Autodesk Fusion 360 part; units mm, degrees
sketch "Sketch1" plane through (0, 0, 0) normal (0, 0, 1) x (1, 0, 0)
  line L0 (38.1, -38.1) -> (-38.1, -38.1)
  line L1 (-38.1, -38.1) -> (-38.1, 38.1)
  line L2 (-38.1, 38.1) -> (38.1, 38.1)
  line L3 (38.1, 38.1) -> (38.1, -38.1)
  line L4 (38.1, -38.1) -> (-38.1, 38.1) construction
  line L5 (-38.1, -38.1) -> (38.1, 38.1) construction
  line L6 (31.75, 31.75) -> (-31.75, 31.75) construction
  line L7 (-31.75, 31.75) -> (-31.75, -31.75) construction
  line L8 (-31.75, -31.75) -> (31.75, -31.75) construction
  line L9 (31.75, -31.75) -> (31.75, 31.75) construction
  line L10 (31.75, 31.75) -> (-31.75, -31.75) construction
  line L11 (-31.75, 31.75) -> (31.75, -31.75) construction
  circle A0 centre (-31.75, 31.75) radius 3
  circle A1 centre (-31.75, -31.75) radius 3
  circle A2 centre (31.75, -31.75) radius 3
  circle A3 centre (31.75, 31.75) radius 3
  circle A4 centre (0, 0) radius 6
  dimension "d1" = 76.2
  dimension "d2" = 76.2
  dimension "d3" = 63.5
  dimension "d4" = 63.5
  dimension "d5" = 6
  dimension "d7" = 360
  dimension "d10" = 12
extrude "Extrude1" add sketch "Sketch1" along normal blind 12.7
sketch "Sketch2" plane through (0, 0, 12.7) normal (0, 0, 1) x (-1, 0, 0)
  circle A0 centre (31.75, -31.75) radius 3
  circle A1 centre (0, 0) radius 6
  circle A2 centre (31.75, 31.75) radius 3
  circle A3 centre (-31.75, -31.75) radius 3
  circle A4 centre (-31.75, 31.75) radius 3
  line L0 (-38.1, -38.1) -> (38.1, -38.1)
  line L1 (38.1, -38.1) -> (38.1, 38.1)
  line L2 (38.1, 38.1) -> (-38.1, 38.1)
  line L3 (-38.1, 38.1) -> (-38.1, -38.1)
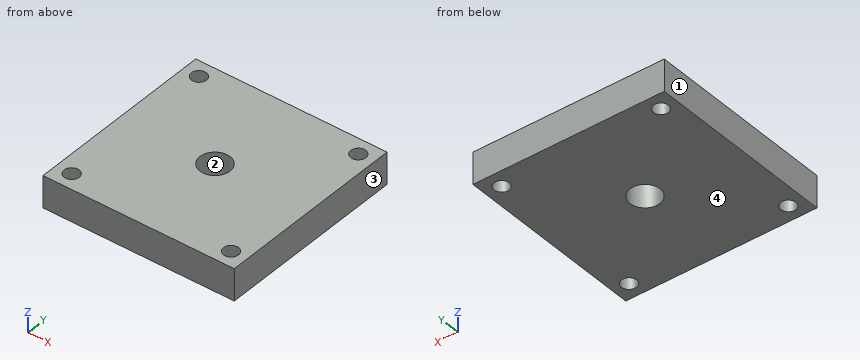
Can you work these out from the model? Positions are in its coordinate system, mm. Face numbers are marked on the shaded views. Give positions to 0.01 mm unless a question says otherwise; leave off trailing zeros. Order: outer loops, then holes, each group sorted by start corner. A loop starts at its lowest first (then second) coordinate and runs counter-clockwise, first axis right, second up. Notation, with made-up numbers: M 0,-11.5 L 58,-11.5 A19 cw 58,22.5 Z; hole C 14,39 d7. An arc over 180 degrees is marked long. Use one line per item in the form item = value. Start each with the question number.
Item 1: If we section it at B-B (y = 0): Write out the boundary of the cut face in (x, z), then the cut area to 3 significant figures.
Item 2: If we section it at A-A (x = -31.75): Write out the boundary of the cut face in (y, z), then the cut area to 3 significant figures.
Item 3: We'd pull the mould along X, two halves only. Please class the marked faces 1, 2, 3 and 4: +X half, -X half, draft (parallel to the pull), parting line (faces both ways), or undercut.
Item 4: If we section it at C-C (z = 8): Write out the boundary of the cut face in (x, y), then the cut area to 3 significant figures.
Item 5: If I drill on line 1 along Y through (x, z) = (-31.75, 2.75); line 2 along X through (y, z) = (-30.5, 7.5); line 3 along Y through (x, z) = (-30, 5.5), over which ranges is the centre line in solid material (lowest first)?
Outcome:
q1.outline = M -38.1,0 L -6,0 L -6,12.7 L -38.1,12.7 Z; M 6,0 L 38.1,0 L 38.1,12.7 L 6,12.7 Z
q1.area = 815 mm2
q2.outline = M -38.1,0 L -34.75,0 L -34.75,12.7 L -38.1,12.7 Z; M -28.75,0 L 28.75,0 L 28.75,12.7 L -28.75,12.7 Z; M 34.75,0 L 38.1,0 L 38.1,12.7 L 34.75,12.7 Z
q2.area = 815 mm2
q3.face_1 = -X half
q3.face_2 = undercut
q3.face_3 = +X half
q3.face_4 = draft
q4.outline = M -38.1,-38.1 L 38.1,-38.1 L 38.1,38.1 L -38.1,38.1 Z; hole C -31.75,-31.75 d6; hole C -31.75,31.75 d6; hole C 0,0 d12; hole C 31.75,-31.75 d6; hole C 31.75,31.75 d6
q4.area = 5,580 mm2
q5.line_1 = -38.1 to -34.75, -28.75 to 28.75, 34.75 to 38.1
q5.line_2 = -38.1 to -34.48, -29.02 to 29.02, 34.48 to 38.1
q5.line_3 = -38.1 to -34.19, -29.31 to 29.31, 34.19 to 38.1
